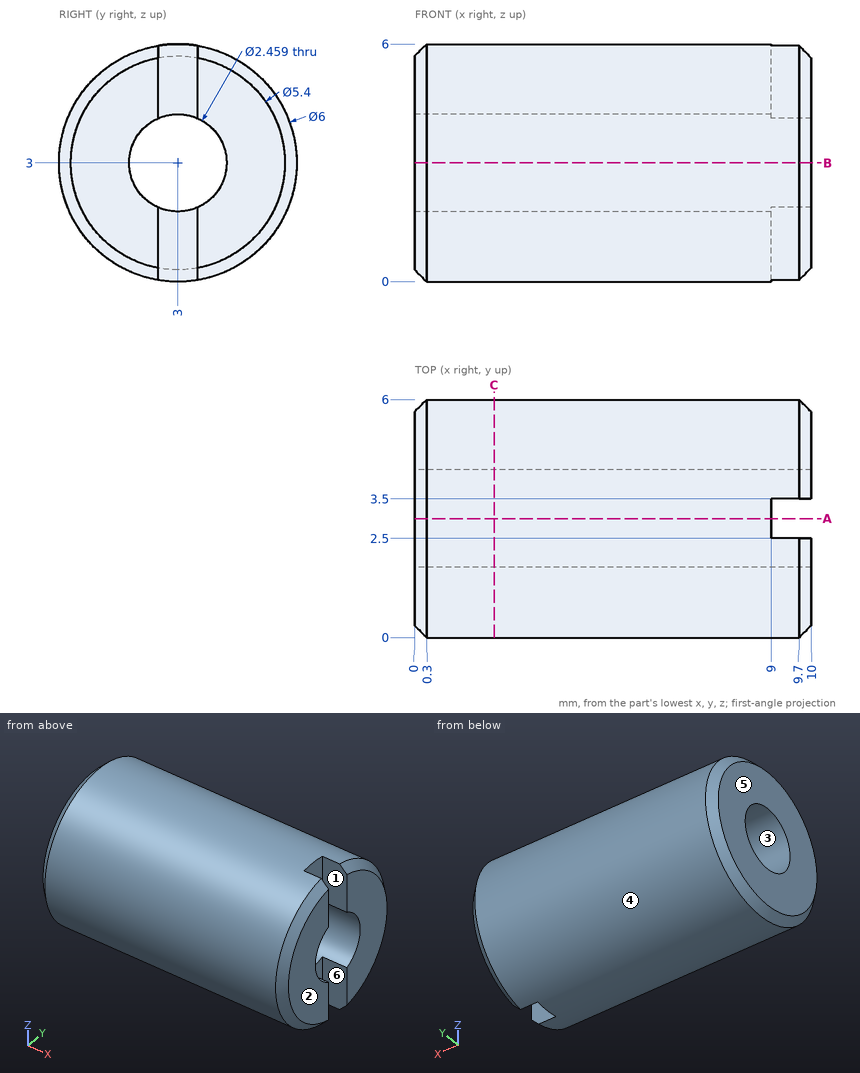
Design review of the part shown in the three views and the two pictorial views. Dimensions are in mm from the part's minimum x, y and z. A direction names the side the tool comes from. Give positions to 0.01 mm unless a question says otherwise; leave off trailing zeros. Loops run counter-clockwise (first coordinate to the right, second up) from the corner with the lowest first, then second, coordinate; pieces in that order, holes last. Notation, with made-up numbers: M 31.5,37 L 90.5,37 A10 ccw 90.5,44 Z; hole C 30.25,84.25 d5. An arc over 180 degrees is marked long. Answer as a JSON object with one key per item and string values.
Item 1: For P1, Ø0.8, axis at x = 9.5, z = 1, coming from the +Y side; P2, Ø1.5, axis at x = 2, y = 1.5, coming from the -Z side; P3, Ø0.5, axis at x = 9.5, z = 1, coming from the -Y side; P4, Ø2, axis at y = 3, z = 3, coming from the +X side, all flat-tipped, find the tip position at first contact; note any pin that passes through.
Output values:
{"P1": "stops at y = 5.54", "P2": "stops at z = 0.1", "P3": "stops at y = 0.56", "P4": "passes through"}
Item 2: Machinability: for the marked faces 5 and 6, which of the approach directions +Z, -Z, +X, -X, +Y, -Y give a long, thin tool a straight path to every point of the face, cutting with its end or side? Answer none if there is none.
Output values:
{"face 5": "+Z, -Z, -X, +Y, -Y", "face 6": "+Z, -Z, +X"}
Item 3: We need section B-B (z = 3). State the section outline as (x, y) points, and give its area (3 significant figures).
Output values:
{"outline": "M 0,0.3 L 0.3,0 L 9.7,0 L 10,0.3 L 10,1.77 L 0,1.77 Z; M 0,4.23 L 10,4.23 L 10,5.7 L 9.7,6 L 0.3,6 L 0,5.7 Z", "area": "35.2 mm2"}
Item 4: We need section C-C (x = 2). State the section outline as (y, z) points, and give its area (3 significant figures).
Output values:
{"outline": "C 3,3 d6; hole C 3,3 d2.46", "area": "23.5 mm2"}
Item 5: Mouldability with a two-part tool opening along Y and no side actions: class the marked faces 1, 2, 3 and 4 as pulls with the +Y half, pulls with the -Y half, needs draft (parallel to the pull), parting line crosses it, or undercut.
Output values:
{"face 1": "undercut", "face 2": "needs draft", "face 3": "undercut", "face 4": "parting line crosses it"}
Item 6: Wall thickness on line 1 along Y through (x, z) = (6.25, 2.5); line 2 along Y through (x, z) = (6.25, 3): over which ranges is each line inside the solid? List them lowest first.
Output values:
{"line 1": "y = 0.04 to 1.88, 4.12 to 5.96", "line 2": "y = 0 to 1.77, 4.23 to 6"}
Item 7: We need section A-A (y = 3). State the section outline as (x, z) points.
Output values:
{"outline": "M 0,0.3 L 0.3,0 L 9,0 L 9,1.77 L 0,1.77 Z; M 0,4.23 L 9,4.23 L 9,6 L 0.3,6 L 0,5.7 Z"}
